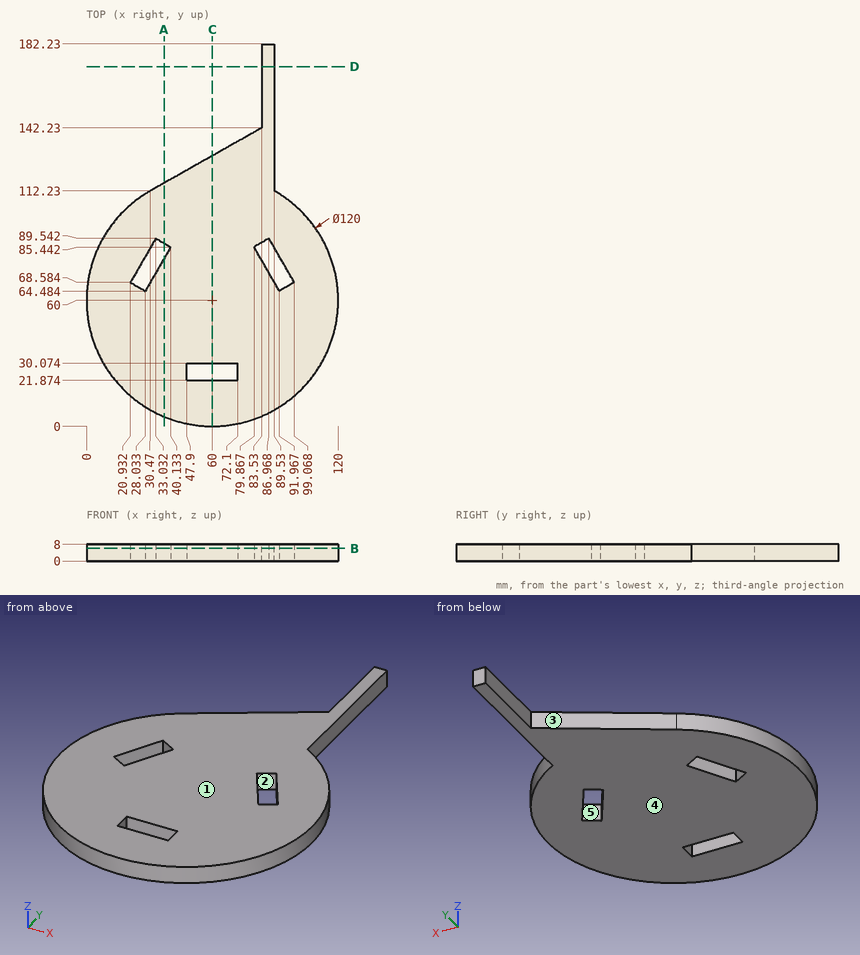
Study the drawing (mm; zero at the part's minimum x, y, z) and answer. A direction names the side the tool comes from. Round coordinates to 2 decimals unless told otherwise and drop trailing zeros. Order: outer loops, then holes, each group sorted by start corner. A loop starts at its lowest first (then second) coordinate and runs counter-clockwise, first axis right, second up. Notation, with made-up numbers: M 14.5,64 L 47.5,64 A26 cw 47.5,78 Z; hole C 46,28 d6. An arc over 180 degrees is marked long. One line per item, written item: value.
Q1. Straight lines are drawn through the part: line 1 (X direction, y = 89, z = 3) (1 decimal); line 2 (X direction, y = 59.5, z = 1.25); line 3 (Y direction, x = 30, z = 1.25). For each, find the intervals that lie inside material, in ascending order.
Derived:
line 1: 7.5 to 32.7, 34 to 86, 87.3 to 112.5
line 2: 0 to 120
line 3: 8.04 to 67.89, 84.29 to 111.96
Q2. Find section A-A on x = 37. Write down the section's boundary in (y, z) (1 decimal), then the cut area to 3 significant figures.
Derived:
outline: M 4.6,0 L 80,0 L 80,8 L 4.6,8 Z; M 87.3,0 L 115.9,0 L 115.9,8 L 87.3,8 Z
area: 833 mm²
Q3. For the marked faces 4 and 5, determine the directions among +Z, -Z, +X, -X, +Y, -Y from which every point of the face is accessible in a straight line to the end or side of a thin tool.
Derived:
face 4: -Z, +X, -X, +Y, -Y
face 5: +Z, -Z
Q4. Flat-ended cylindrical pins translate along their axes: pin 1 (2.5 mm diameter, centred on y = 172, z = 3.5, fed in from -X); pin 2 (1 mm diameter, centred on x = 57.5, z = 3.5, fed in from +Y) (1 decimal); pin 3 (1 mm diameter, centred on y = 57.5, z = 6.5, fed in from -X). Find the tip coordinate at first contact, or state that the pin passes through.
Derived:
pin 1: x = 83.53
pin 2: y = 127.8
pin 3: x = 0.03
Q5. Find section D-D on y = 171.5. Write down the section's boundary in (x, z).
Derived:
outline: M 83.53,0 L 89.53,0 L 89.53,8 L 83.53,8 Z
Q6. Find section B-B on z = 6. Write down the section's boundary in (x, y).
Derived:
outline: M 30.47,112.23 A60 ccw long 89.53,112.23 L 89.53,182.23 L 83.53,182.23 L 83.53,142.23 Z; hole M 20.93,68.58 L 28.03,64.48 L 40.13,85.44 L 33.03,89.54 Z; hole M 47.9,21.87 L 72.1,21.87 L 72.1,30.07 L 47.9,30.07 Z; hole M 79.87,85.44 L 91.97,64.48 L 99.07,68.58 L 86.97,89.54 Z
Q7. Determine the mould class of the marked faces 1, 2 and 3 for opening direction X: released by +X, released by -X, zero draft, split by the parting line, or undercut.
Derived:
face 1: zero draft
face 2: undercut
face 3: released by -X
Q8. Find section C-C on x = 60. Write down the section's boundary in (y, z).
Derived:
outline: M 0,0 L 21.87,0 L 21.87,8 L 0,8 Z; M 30.07,0 L 128.93,0 L 128.93,8 L 30.07,8 Z
